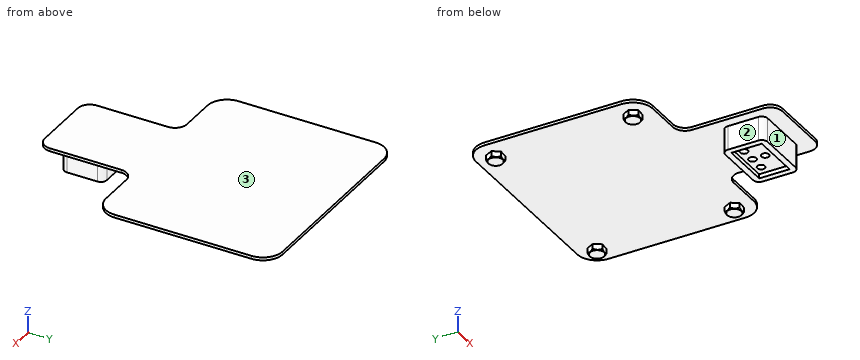
from build123d import *

# Parameters (mm, degrees)
BOSS_EXTRUDE1_DEPTH = 5
SKETCH2_R           = 9
CUT_EXTRUDE1_DEPTH  = 75
BOSS_EXTRUDE2_DEPTH = 15
SKETCH4_R           = 18.116170111
SKETCH4_R_2         = 11.683917043
CUT_EXTRUDE2_DEPTH  = 15
CUT_EXTRUDE2_TAPER  = 45
SKETCH5_W           = 100.933414707
SKETCH5_H           = 70.54527083
BOSS_EXTRUDE3_DEPTH = 40
FILLET1_R           = 10
SKETCH6_W           = 80.933414707
SKETCH6_H           = 50.54527083
CUT_EXTRUDE3_DEPTH  = 7
SKETCH7_R           = 6.405339055
CUT_EXTRUDE4_DEPTH  = 22


with BuildPart() as part:
    # Sketch1 → Boss-Extrude1 (new body)
    with BuildSketch(Plane.XY):
        with BuildLine():
            Line((-147.184574627, 293.941978101), (147.184574627, 293.941978101))
            ThreePointArc((147.184574627, 293.941978101), (170.33130349, 284.354289081), (179.91899251, 261.207560218))
            Line((179.91899251, 261.207560218), (179.91899251, 32.734417883))
            ThreePointArc((179.91899251, 32.734417883), (170.33130349, 9.58768902), (147.184574627, 0))
            Line((147.184574627, 0), (87.922065379, 0))
            ThreePointArc((87.922065379, 0), (73.779929755, -5.857864376), (67.922065379, -20))
            Line((67.922065379, -20), (67.922065379, -138.690071177))
            ThreePointArc((67.922065379, -138.690071177), (62.064201003, -152.832206801), (47.922065379, -158.690071177))
            Line((47.922065379, -158.690071177), (-47.922065379, -158.690071177))
            ThreePointArc((-47.922065379, -158.690071177), (-62.064201003, -152.832206801), (-67.922065379, -138.690071177))
            Line((-67.922065379, -138.690071177), (-67.922065379, -20))
            ThreePointArc((-67.922065379, -20), (-73.779929755, -5.857864376), (-87.922065379, 0))
            Line((-87.922065379, 0), (-147.184574627, 0))
            ThreePointArc((-147.184574627, 0), (-170.33130349, 9.58768902), (-179.91899251, 32.734417883))
            Line((-179.91899251, 32.734417883), (-179.91899251, 261.207560218))
            ThreePointArc((-179.91899251, 261.207560218), (-170.33130349, 284.354289081), (-147.184574627, 293.941978101))
        make_face()
    extrude(amount=BOSS_EXTRUDE1_DEPTH)

    # Sketch2 → Cut-Extrude1 (cut)
    with BuildSketch(Plane.XY.offset(5)):
        with Locations((-147.184574627, 261.207560218)):
            Circle(SKETCH2_R)
        with Locations((147.184574627, 261.207560218)):
            Circle(SKETCH2_R)
        with Locations((147.184574627, 32.734417883)):
            Circle(SKETCH2_R)
        with Locations((-147.184574627, 32.734417883)):
            Circle(SKETCH2_R)
    extrude(amount=-CUT_EXTRUDE1_DEPTH, mode=Mode.SUBTRACT)

    # Sketch3 → Boss-Extrude2 (add)
    with BuildSketch(Plane.XY.offset(5)):
        Polygon((139.58276715, 272.953720991), (133.211197263, 260.497282214), (140.81300474, 248.751121442), (154.786382105, 249.461399446), (161.157951992, 261.917838222), (153.556144514, 273.663998995), align=None)
        Polygon((-140.81300474, 273.663998995), (-154.786382105, 272.953720991), (-161.157951992, 260.497282214), (-153.556144514, 248.751121442), (-139.58276715, 249.461399446), (-133.211197263, 261.917838222), align=None)
        Polygon((139.58276715, 44.480578655), (133.211197263, 32.024139879), (140.81300474, 20.277979107), (154.786382105, 20.988257111), (161.157951992, 33.444695887), (153.556144514, 45.190856659), align=None)
        Polygon((-154.786382105, 44.480578655), (-161.157951992, 32.024139879), (-153.556144514, 20.277979107), (-139.58276715, 20.988257111), (-133.211197263, 33.444695887), (-140.81300474, 45.190856659), align=None)
    extrude(amount=-BOSS_EXTRUDE2_DEPTH)

    # Sketch4 → Cut-Extrude2 (cut)
    # profile 1 of 4: a face of its own
    with BuildSketch(Plane(origin=(0, 0, -10), x_dir=(-1, 0, 0), z_dir=(0, 0, -1))):
        with Locations((-147.184574627, 261.207560218)):
            Circle(SKETCH4_R)
        with Locations((-147.184574627, 261.207560218)):
            Circle(SKETCH4_R_2, mode=Mode.SUBTRACT)
    # profile 2 of 4: a face of its own
    with BuildSketch(Plane(origin=(0, 0, -10), x_dir=(-1, 0, 0), z_dir=(0, 0, -1))):
        with Locations((-147.184574627, 32.734417883)):
            Circle(SKETCH4_R)
        with Locations((-147.184574627, 32.734417883)):
            Circle(SKETCH4_R_2, mode=Mode.SUBTRACT)
    # profile 3 of 4: a face of its own
    with BuildSketch(Plane(origin=(0, 0, -10), x_dir=(-1, 0, 0), z_dir=(0, 0, -1))):
        with Locations((147.184574627, 32.734417883)):
            Circle(SKETCH4_R)
        with Locations((147.184574627, 32.734417883)):
            Circle(SKETCH4_R_2, mode=Mode.SUBTRACT)
    # profile 4 of 4: a face of its own
    with BuildSketch(Plane(origin=(0, 0, -10), x_dir=(-1, 0, 0), z_dir=(0, 0, -1))):
        with Locations((147.184574627, 261.207560218)):
            Circle(SKETCH4_R)
        with Locations((147.184574627, 261.207560218)):
            Circle(SKETCH4_R_2, mode=Mode.SUBTRACT)
    extrude(amount=-CUT_EXTRUDE2_DEPTH, taper=CUT_EXTRUDE2_TAPER, mode=Mode.SUBTRACT)

    # Sketch5 → Boss-Extrude3 (add)
    with BuildSketch(Plane(origin=(0, 0, 0), x_dir=(-1, 0, 0), z_dir=(0, 0, -1))):
        with Locations((0.645780789, -95.485224261)):
            Rectangle(SKETCH5_W, SKETCH5_H)
    extrude(amount=BOSS_EXTRUDE3_DEPTH)

    # Fillet1
    fillet1_edges = [part.edges().sort_by_distance(p)[0] for p in [
        (49.820926565, -60.212588846, -20),
        (49.820926565, -130.757859676, -20),
        (-51.112488142, -130.757859676, -20),
        (-51.112488142, -60.212588846, -20),
    ]]
    fillet(fillet1_edges, radius=FILLET1_R)

    # Sketch6 → Cut-Extrude3 (cut)
    with BuildSketch(Plane(origin=(0, 0, -40), x_dir=(-1, 0, 0), z_dir=(0, 0, -1))):
        with Locations((0.645780789, -95.485224261)):
            Rectangle(SKETCH6_W, SKETCH6_H)
    extrude(amount=-CUT_EXTRUDE3_DEPTH, mode=Mode.SUBTRACT)

    # Sketch7 → Cut-Extrude4 (cut)
    with BuildSketch(Plane(origin=(0, 0, -33), x_dir=(-1, 0, 0), z_dir=(0, 0, -1))):
        with Locations((-24.146994076, -82.382499347)):
            Circle(SKETCH7_R)
        with Locations((0.645780789, -82.382499347)):
            Circle(SKETCH7_R)
        with Locations((0.645780789, -103.378848644)):
            Circle(SKETCH7_R)
        with Locations((25.493027066, -82.382499347)):
            Circle(SKETCH7_R)
    extrude(amount=-CUT_EXTRUDE4_DEPTH, mode=Mode.SUBTRACT)


solid = part.part
Check sheet for the modelled part. Datum: model origin and axes. Units: mm. Face numbers are marked on the shaded views. A direction names the side the tool comes from. Coordinates: 2 decimals unless noted, no trailing zeros. Loops run counter-clockwise (first coordinate to the right, second up) from the corner with the lowest first, then second, coordinate; pieces in that order, holes last. Notation, with made-up numbers: (-33.5, 77) -> (17.5, 77) arc R20 cw to (17.5, 106) -> close; hole circle Ø4 at (64, -9.75). An arc over 180 degrees is marked (long way). Answer in a Markdown table with one row per item.
1. Material ranges on line 1 along X through (y, z) = (-130.5, 2); line 2 along Y through (x, z) = (31.5, -14.5); line 3 along Y through (x, z) = (-135.5, -7.5), recorded low to high. Write a range as [from, to].
Check values:
| item | result |
|---|---|
| line 1 | x = [-67.92, 67.92] |
| line 2 | y = [-130.76, -60.21] |
| line 3 | y = [28.97, 36.98], [257.44, 265.45] |
2. Access from +Z, -Z, +X, -X, +Y, -Y to the whole of each face (thin tool, end or side, straight path). Record for the marked faces 1, 2 and 3.
Check values:
| item | result |
|---|---|
| face 1 | -Z, +X, -X, -Y |
| face 2 | -Z, -X, +Y, -Y |
| face 3 | +Z, +X, -X, +Y, -Y |
3. Sectioned sample at B-B, the plane y = -46. Record the boundary of the cut face in (x, z), then the cut area to 3 significant figures.
Check values:
| item | result |
|---|---|
| outline | (-67.92, 0) -> (67.92, 0) -> (67.92, 5) -> (-67.92, 5) -> close |
| area | 679 mm2 |
4. Sectioned sample at C-C, the plane x = 121. Record the boundary of the cut face in (y, z), then the cut area to 3 significant figures.
Check values:
| item | result |
|---|---|
| outline | (0, 0) -> (293.94, 0) -> (293.94, 5) -> (0, 5) -> close |
| area | 1,470 mm2 |
5. Go/stop test with flat-tipped pins: pin 1 (4 mm diameter, centred on x = -3.5, y = -103, fed in from -Z); pin 2 (5 mm diameter, centred on y = -89.5, z = -3.5, fed in from -X); pin 3 (7.5 mm diameter, centred on x = 17.5, z = -35.5, fed in from -Y). Record where each tip stops, or that it passes through.
Check values:
| item | result |
|---|---|
| pin 1 | stops at z = -11 |
| pin 2 | stops at x = -51.11 |
| pin 3 | stops at y = -130.76 |
6. Sectioned sample at A-A, the plane x = -13.5. Record the boundary of the cut face in (y, z).
Check values:
| item | result |
|---|---|
| outline | (-158.69, 0) -> (-130.76, 0) -> (-130.76, -40) -> (-120.76, -40) -> (-120.76, -33) -> (-70.21, -33) -> (-70.21, -40) -> (-60.21, -40) -> (-60.21, 0) -> (293.94, 0) -> (293.94, 5) -> (-158.69, 5) -> close |
